Work out the finished part from the listing and answer in its coordinate system (mm). A direction names the side the tool comes from. Coordinates: 2 decimals unless noted, no trailing zeros. Order: outer loops, then holes, each group sorted by start corner. A loop starts at its lowest first (then second) coordinate and runs counter-clockwise, first axis right, second up.
1. A flat-ended cylindrical pin translates along its axis: pin 1 Ø1 at (y, z) = (1, 1) entering from -X. Find the tip coordinate at first contact, or state that the pin passes through.
2. A tool of negligible diameter and unlimited length cuts with its end or side. For faces 1 (the flat face through (2, 2, 3)), 2 (the flat face through (3, 4, 1)), from which of +Z, -Z, +X, -X, +Y, -Y can it reach the whole face along a straight path? Write none if from no direction.
3. The part is cut by section A-A, the plane y = 1.3. Give the vertices of the cut face in (x, z), then the cut area to 3 significant figures.
4. The part is cut by section D-D, the plane z = 2.8. Give the vertices of the cut face in (x, y), then the cut area to 3 significant figures.
5. Find the intervals of material crossed by probe 1 along X at (y, z) = (4.55, 3); probe 2 along Y at (x, z) = (4.6, 0.75); probe 3 along X at (y, z) = (1.9, 1.6), in increasing order.
6. The part is cut by section C-C, the plane z = 0.9. Give the vertices of the cut face in (x, y).
```python
from build123d import *

# Parameters (mm, degrees)
BOSS_EXTRUDE1_DEPTH = 2
SKETCH2_W           = 6
SKETCH2_H           = 5.001068762
BOSS_EXTRUDE2_DEPTH = 2
CHAMFER1_SIZE       = 1
CHAMFER1_SIZE2      = 2
CUT_EXTRUDE2_DEPTH  = 2
CUT_EXTRUDE3_DEPTH  = 2


with BuildPart() as part:
    # Sketch1 → Boss-Extrude1 (new body)
    with BuildSketch(Plane.XY):
        Polygon((0, 0), (6, 0), (6, 5), (2, 5), (0, 5), (0, 3), align=None)
    extrude(amount=BOSS_EXTRUDE1_DEPTH)

    # Sketch2 → Boss-Extrude2 (add)
    with BuildSketch(Plane.XY.offset(2)):
        with Locations((3, 2.500534381)):
            Rectangle(SKETCH2_W, SKETCH2_H)
    extrude(amount=BOSS_EXTRUDE2_DEPTH)

    # Chamfer1
    chamfer1_edges = [part.edges().sort_by_distance(p)[0] for p in [
        (3, 5.001068762, 4),
    ]]
    chamfer1_side = [part.faces().sort_by_distance(p)[0] for p in [
        (3, 5.001068762, 3),
    ]]
    chamfer(chamfer1_edges, length=CHAMFER1_SIZE, length2=CHAMFER1_SIZE2, reference=chamfer1_side[0])

    # 3DSketch1 → Cut-Extrude2 (cut, along a direction that is not the sketch's normal)
    with BuildSketch(Plane(origin=(2, 5.001068762, 3), x_dir=(0.36508333931807946, -0.9129034418767683, 0.18254166965903973), z_dir=(0.447213595499958, 0, -0.894427190999916))):
        Polygon((0, 0), (2.738515232, -1.224962989), (5.478201234, 0), (3.652784538, 4.082628306), (-0.912708348, 2.041314153), align=None)
    extrude(amount=-CUT_EXTRUDE2_DEPTH, dir=(0, 0, -1), mode=Mode.SUBTRACT)

    # Sketch4 → Cut-Extrude3 (cut)
    with BuildSketch(Plane(origin=(0, 0, 0), x_dir=(-1, 0, 0), z_dir=(0, 0, -1))):
        Polygon((0, 5.000534381), (-2, 5.001068762), (-4, 3.001068762), (-4, 0), (0, 0), align=None)
    extrude(amount=-CUT_EXTRUDE3_DEPTH, mode=Mode.SUBTRACT)


solid = part.part
```
Geometry says:
1. pin 1: stops at x = 4
2. face 1: +Z, -X, +Y, -Y
2. face 2: -Z, -X, -Y
3. outline: (0, 2) - (4, 2) - (4, 0) - (6, 0) - (6, 4) - (4, 4) - close
3. area: 12.0 mm2
4. outline: (1.6, 0) - (6, 0) - (6, 5) - (1.6, 5) - close
4. area: 22.0 mm2
5. probe 1: x = 2 to 6
5. probe 2: y = 0 to 5
5. probe 3: x = 4 to 6
6. outline: (2, 5) - (4, 3) - (4, 0) - (6, 0) - (6, 5) - close
